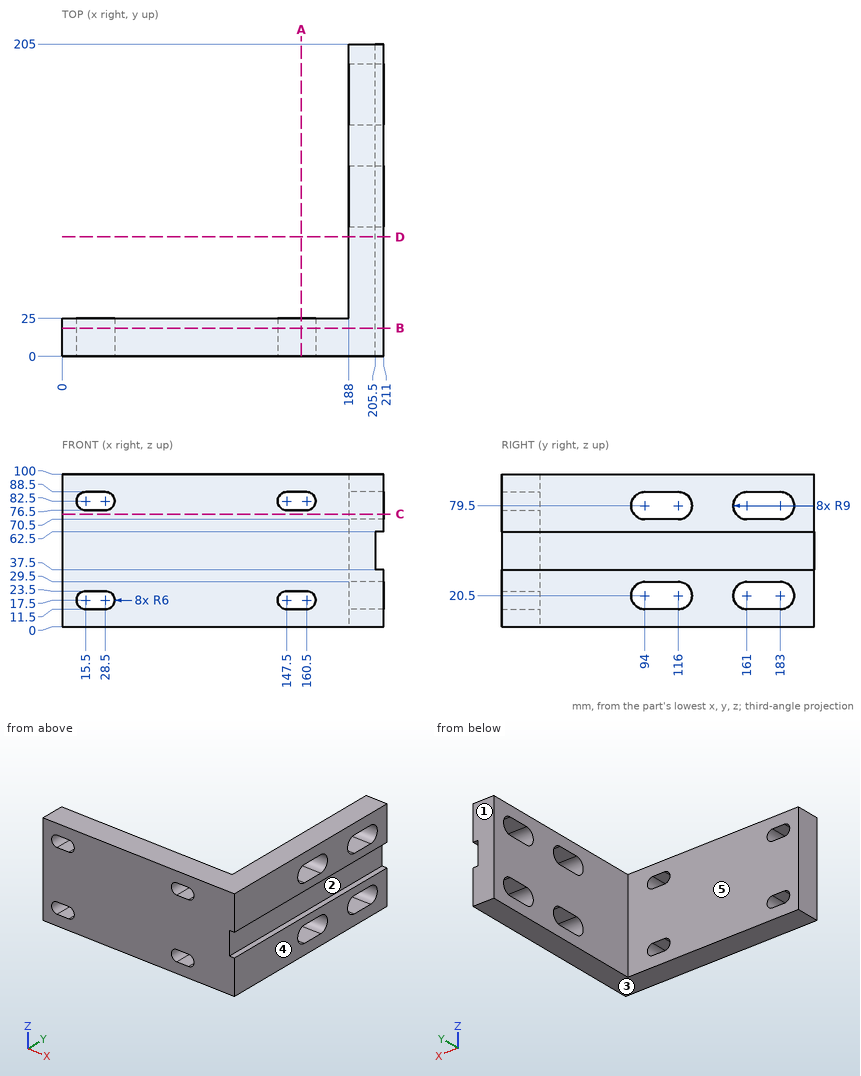
Input: dimensioned drawing with shaded views. Units: mm. Origin: part minimum x, y, z. A direction names the side the tool comes from. Coordinates: 2 decimals unless noted, no trailing zeros. Loops run counter-clockwise (first coordinate to the right, second up) from the corner with the lowest first, then second, coordinate; pieces in that order, holes last. Notation, with made-up numbers: (-17.5, 26) -> (5.5, 26) arc R24 ccw to (5.5, 37) -> close; hole circle Ø6 at (6, 57.5). An arc over 180 degrees is marked (long way). Use a Markdown table: item, result. Add a question column.
(1) Section query B-B, the plane y = 18.5. Return loops of the section in (x, z).
(2) Section query A-A, the plane x = 157. Return loops of the section in (y, z).
(3) Mould query, pull axis Z, two halves, no side actions, for the marked faces 1, 2 and 3. Classes: pulls with the +Z half, pulls with the -Z half, needs draft (parallel to the pull), parting line crosses it, or undercut.
(4) Section query D-D, the plane y = 78.5. Return loops of the section in (x, z).
(5) Access query for the marked faces 4 and 5. Directions: +Z, -Z, +X, -X, +Y, -Y. A direction counts if a zero-diameter tool reaches every point of the face in a straight line with its end or side. Return the directions, or none.
(6) Section query C-C, the plane z = 74. Return loops of the section in (x, y).
(7) Line query: line 1 along Z through (x, y) = (195.5, 111.5); line 2 along Z through (x, y) = (200, 121); line 3 along X through (y, z) = (15, 16.5). Output: solid intervals per line, ascending.
(8) Pin query (flat end, axial travel): pin 1 Ø3 at (x, z) = (76.5, 51) entering from +Y; pin 2 Ø4 at (y, z) = (79, 50) entering from -X. Return the tip coordinate at first contact, or that it passes through.
Answer:
| question | item | result |
|---|---|---|
| 1 | outline | (0, 0) -> (211, 0) -> (211, 37.5) -> (205.5, 37.5) -> (205.5, 62.5) -> (211, 62.5) -> (211, 100) -> (0, 100) -> close; hole (15.5, 11.5) -> (28.5, 11.5) arc R6 ccw to (28.5, 23.5) -> (15.5, 23.5) arc R6 ccw to start; hole (15.5, 76.5) -> (28.5, 76.5) arc R6 ccw to (28.5, 88.5) -> (15.5, 88.5) arc R6 ccw to start; hole (147.5, 11.5) -> (160.5, 11.5) arc R6 ccw to (160.5, 23.5) -> (147.5, 23.5) arc R6 ccw to start; hole (147.5, 76.5) -> (160.5, 76.5) arc R6 ccw to (160.5, 88.5) -> (147.5, 88.5) arc R6 ccw to start |
| 2 | outline | (0, 0) -> (25, 0) -> (25, 11.5) -> (0, 11.5) -> close; (0, 23.5) -> (25, 23.5) -> (25, 76.5) -> (0, 76.5) -> close; (0, 88.5) -> (25, 88.5) -> (25, 100) -> (0, 100) -> close |
| 3 | face 1 | needs draft |
| 3 | face 2 | undercut |
| 3 | face 3 | pulls with the -Z half |
| 4 | outline | (188, 0) -> (211, 0) -> (211, 37.5) -> (205.5, 37.5) -> (205.5, 62.5) -> (211, 62.5) -> (211, 100) -> (188, 100) -> close |
| 5 | face 4 | +Z, -Z, +X, +Y, -Y |
| 5 | face 5 | +Z, -Z, -X, +Y |
| 6 | outline | (0, 0) -> (211, 0) -> (211, 86.88) -> (188, 86.88) -> (188, 25) -> (0, 25) -> close; (188, 123.12) -> (211, 123.12) -> (211, 153.88) -> (188, 153.88) -> close; (188, 190.12) -> (211, 190.12) -> (211, 205) -> (188, 205) -> close |
| 7 | line 1 | z = 0 to 11.5, 29.5 to 70.5, 88.5 to 100 |
| 7 | line 2 | z = 0 to 13.02, 27.98 to 72.02, 86.98 to 100 |
| 7 | line 3 | x = 0 to 9.58, 34.42 to 141.58, 166.42 to 211 |
| 8 | pin 1 | stops at y = 25 |
| 8 | pin 2 | stops at x = 188 |
